Autodesk Inventor part; units mm, degrees
ref_plane "YZ Plane" through (0, 0, 0) normal (1, 0, 0) x (0, 1, 0)
ref_plane "XZ Plane" through (0, 0, 0) normal (0, 1, 0) x (-1, 0, 0)
ref_plane "XY Plane" through (0, 0, 0) normal (0, 0, 1) x (1, 0, 0)
sketch "Sketch2" plane through (0, 0, 0) normal (0, 0, 1) x (1, 0, 0)
  line L0 (0, 0) -> (0, 2.5)
  line L1 (0, 2.5) -> (9, 2.5)
  line L2 (9, 2.5) -> (9, 4)
  line L3 (9, 4) -> (51, 4)
  line L4 (51, 4) -> (51, 2.5)
  line L5 (51, 2.5) -> (59, 2.5)
  line L6 (59, 2.5) -> (59, 0)
  line L7 (59, 0) -> (0, 0)
  dimension "d0" = 5
  dimension "d1" = 8
  dimension "d2" = 9
  dimension "d3" = 8
  dimension "d4" = 42
revolve "Revolution1" add sketch "Sketch2" angle 360 about axis through (59, 0, 0) along (-1, 0, 0)
thread "Thread1"
thread "Thread2"
properties part number "46"
Input: part model. Units: mm. Frame: model coordinates. A direction names the side the tool comes from. Give positions to 0.01 mm unless a question says otherwise; leave off trailing zeros. Order: outer loops, then holes, each group sorted by start corner. A loop starts at its lowest first (then second) coordinate and runs counter-clockwise, first axis right, second up. Notation, with made-up numbers: (8, 17) - (14, 17) arc R27 cw to (14, 38) - close; hole circle Ø9 at (44, 6). An arc over 180 degrees is marked (long way). Use a Markdown table: item, result.
(1) Line query: line 1 (X direction, y = -2, z = 2.5); line 2 (Z direction, x = 50, y = 0.25); line 3 (Z direction, x = 33, y = -2.25). Output: solid intervals per line, ascending. Write a range as from..to.
Computed values:
| item | result |
|---|---|
| line 1 | x = 9..51 |
| line 2 | z = -3.99..3.99 |
| line 3 | z = -3.31..3.31 |
(2) Pin query (flat end, axial travel): pin 1 (1.5 mm diameter, centred on x = 11, z = -1, fed in from -Y); pin 2 (1 mm diameter, centred on x = 43, y = 1.5, fed in from -Z); pin 3 (1.5 mm diameter, centred on x = 50.5, y = -1, fed in from -Z). Return the tip coordinate at first contact, or that it passes through.
Computed values:
| item | result |
|---|---|
| pin 1 | stops at y = -3.99 |
| pin 2 | stops at z = -3.87 |
| pin 3 | stops at z = -3.99 |
(3) Section query A-A (z = 0). Output: boundary loops of the cut face in (x, y).
Computed values:
| item | result |
|---|---|
| outline | (0, -2.5) - (9, -2.5) - (9, -4) - (51, -4) - (51, -2.5) - (59, -2.5) - (59, 2.5) - (51, 2.5) - (51, 4) - (9, 4) - (9, 2.5) - (0, 2.5) - close |
(4) Section query C-C (x = 38.5). Output: boundary loops of the cut face in (y, z).
Computed values:
| item | result |
|---|---|
| outline | circle Ø8 at (0, 0) |
(5) Access query for faces 1 (the cylindrical face through (30.294, -0.867, -3.905)), 2 (the flat face through (9, 2, -2)), 3 (the cylindrical face through (55.06, -0.54, -2.44)). Directions: +Z, -Z, +X, -X, +Y, -Y. A direction counts if a zero-diameter tool reaches every point of the face in a straight line with its end or side. Return the directions, or none.
Computed values:
| item | result |
|---|---|
| face 1 | +X, -X |
| face 2 | -X |
| face 3 | +X |
(6) Section query D-D (z = -3.5). Output: boundary loops of the cut face in (x, y), then the cut area to 3 significant figures.
Computed values:
| item | result |
|---|---|
| outline | (9, -1.94) - (51, -1.94) - (51, 1.94) - (9, 1.94) - close |
| area | 163 mm2 |
